from build123d import *

# Parameters (mm, degrees)
ESQUISSE1_R        = 2
BOSS_EXTRU_1_DEPTH = 5
ESQUISSE2_R        = 4.5
BOSS_EXTRU_2_DEPTH = 3
CONG_1_R           = 2


with BuildPart() as part:
    # Esquisse1 → Boss.-Extru.1 (new body)
    with BuildSketch(Plane.XY):
        Circle(ESQUISSE1_R)
    extrude(amount=BOSS_EXTRU_1_DEPTH)

    # Esquisse2 → Boss.-Extru.2 (add)
    with BuildSketch(Plane.XY):
        Circle(ESQUISSE2_R)
        Polygon((-1.718731116, -0.115769453), (-1.718731116, 0.115769453), (-0.115769453, 0.115769453), (-0.115769453, 1.718731116), (0.115769453, 1.718731116), (0.115769453, 0.115769453), (1.718731116, 0.115769453), (1.718731116, -0.115769453), (0.115769453, -0.115769453), (0.115769453, -1.718731116), (-0.115769453, -1.718731116), (-0.115769453, -0.115769453), align=None, mode=Mode.SUBTRACT)
    extrude(amount=-BOSS_EXTRU_2_DEPTH)

    # Congé1
    cong_1_edges = [part.edges().sort_by_distance(p)[0] for p in [
        (-4.5, 0, -3),
    ]]
    fillet(cong_1_edges, radius=CONG_1_R)


solid = part.part
Geometry check sheet. Reference: the model listing, model coordinates, mm. A direction names the side the tool comes from. Coordinates: 2 decimals unless noted, no trailing zeros. Order: outer loops, then holes, each group sorted by start corner. A loop starts at its lowest first (then second) coordinate and runs counter-clockwise, first axis right, second up. Notation, with made-up numbers: (61, 86.5) - (112, 86.5) arc R9 cw to (112, 102.5) - close; hole circle Ø3 at (83.5, 8.5). An arc over 180 degrees is marked (long way). Answer in a Markdown table with one row per item. Add a question column.
1) Cross-section at A-A, the plane z = -0.5. Record the cut outline in (x, y), then the cut area to 3 significant figures.
2) Material ranges on line 1 along Z through (x, y) = (2, 1.5); line 2 along Y through (x, z) = (-0.75, -2.25); line 3 along Y through (x, z) = (-3, -1), recorded low to high. Write a range as [from, to].
3) Cross-section at C-C, the plane z = 2. Record the cut outline in (x, y).
4) Gauge pin test, flat ends, axial feed: P1, Ø1.5, axis at x = 2, z = -0.5, coming from the -Y side; P2, Ø0.5, axis at y = -1, z = -1, coming from the +X side; P3, Ø0.8, axis at y = -1, z = -2, coming from the -X side. Record the tip position at first contact, or that the pin passes through.
5) Release check for a two-part mould opening along Y. For faces 4 (the flat face through (0.116, 1, -1)), 5 (the cylindrical face through (0, -2, 2)), 6 (the flat face through (0, 0, 5)) record: +Y half, -Y half, draft (parallel to the pull), parting line (faces both ways), or undercut.
6) Cross-section at B-B, the plane z = -2. Record the cut outline in (x, y), then the cut area to 3 significant figures.
7) Set-up check for faces 1 (the flat face through (1, 0.116, -1)), 2 (the flat face through (2, -1, 0)), 3 (the flat face through (1, -1, -3)): record each of +Z, -Z, +X, -X, +Y, -Y from which the full face is reachable in a straight line by a thin tool's end or side.
Check result:
| question | item | result |
|---|---|---|
| 1 | outline | circle Ø9 at (0, 0); hole (-1.72, -0.12) - (-0.12, -0.12) - (-0.12, -1.72) - (0.12, -1.72) - (0.12, -0.12) - (1.72, -0.12) - (1.72, 0.12) - (0.12, 0.12) - (0.12, 1.72) - (-0.12, 1.72) - (-0.12, 0.12) - (-1.72, 0.12) - close |
| 1 | area | 62.1 mm² |
| 2 | line 1 | z = [-3, 0] |
| 2 | line 2 | y = [-3.99, -0.12], [0.12, 3.99] |
| 2 | line 3 | y = [-3.35, 3.35] |
| 3 | outline | circle Ø4 at (0, 0) |
| 4 | P1 | stops at y = -4.32 |
| 4 | P2 | stops at x = 4.44 |
| 4 | P3 | stops at x = -4.32 |
| 5 | face 4 | undercut |
| 5 | face 5 | parting line |
| 5 | face 6 | draft |
| 6 | outline | circle Ø8.46 at (0, 0); hole (-1.72, -0.12) - (-0.12, -0.12) - (-0.12, -1.72) - (0.12, -1.72) - (0.12, -0.12) - (1.72, -0.12) - (1.72, 0.12) - (0.12, 0.12) - (0.12, 1.72) - (-0.12, 1.72) - (-0.12, 0.12) - (-1.72, 0.12) - close |
| 6 | area | 54.7 mm² |
| 7 | face 1 | -Z |
| 7 | face 2 | +Z |
| 7 | face 3 | -Z, +X, -X, +Y, -Y |
